```python
from build123d import *

# Parameters (mm, degrees)
F1_DEPTH = 60
F5_D     = 7
F5_DEPTH = 50
F5_TIP   = 2.1030121666
F7_DEPTH = 4.5
F9_DEPTH = 4.5
F10_R    = 1


with BuildPart() as f1:
    # F0 (on Front) → F1 (new body)
    with BuildSketch(Plane.XZ):
        with BuildLine():
            Line((-10, 10), (-10, 0))
            Line((-10, 0), (-7.5, 0))
            Line((-7.5, 0), (-7.5, 5))
            Line((-7.5, 5), (-2.5, 5))
            Line((-2.5, 5), (-2.5, 0))
            Line((-2.5, 0), (2.5, 0))
            Line((2.5, 0), (2.5, 5))
            Line((2.5, 5), (7.5, 5))
            Line((7.5, 5), (7.5, 0))
            Line((7.5, 0), (10, 0))
            Line((10, 0), (10, 10))
            ThreePointArc((10, 10), (0, 20), (-10, 10))
        make_face()
    extrude(amount=-F1_DEPTH)

    # F2 (on Right) → F3 (revolve)
    with BuildSketch(Plane.YZ):
        with BuildLine():
            Line((0, 5), (0, 15))
            ThreePointArc((0, 15), (-5, 10), (0, 5))
        make_face()
    revolve(axis=Axis((0, 0, 10), (0, 0, -1)))

    # F5
    with Locations(Plane(origin=(0, 60, 0), x_dir=(-1, 0, 0), z_dir=(0, 1, 0))):
        with Locations((0, 10)):
            Hole(F5_D / 2, depth=F5_DEPTH)
            with Locations((0, 0, -(F5_DEPTH + F5_TIP / 2))):  # 118° drill point
                Cone(0, F5_D / 2, F5_TIP, mode=Mode.SUBTRACT)

    # F6 (on face) → F7 (join)
    with BuildSketch(Plane.YZ.offset(10)):
        Polygon((45, 0), (60, 0), (48, 10), (45, 10), align=None)
    extrude(amount=F7_DEPTH)

    # F8 (on face) → F9 (join)
    with BuildSketch(Plane(origin=(-10, 0, 0), x_dir=(0, -1, 0), z_dir=(-1, 0, 0))):
        Polygon((-48, 10), (-60, 0), (-45, 0), (-45, 10), align=None)
    extrude(amount=F9_DEPTH)

    # F10
    f10_edges = [f1.edges().sort_by_distance(p)[0] for p in [
        (12.25, 45, 10),
        (12.25, 48, 10),
        (-12.25, 45, 10),
        (-12.25, 48, 10),
    ]]
    fillet(f10_edges, radius=F10_R)


solid = f1.part
```
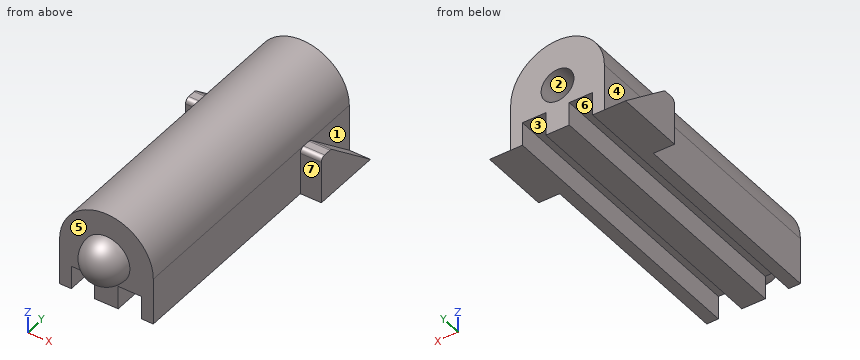
Could you check a few things on this model? Use its own coordinates, in mm. Face numbers are marked on the shaded views. A direction names the side the tool comes from. Coordinates: 2 decimals unless noted, no trailing zeros. Write each loop counter-clockwise with the first axis right and the second up, starting at its lowest first coordinate (ties: lowest second). Pieces come first, ordered by that corner, then holes. Notation, with made-up numbers: (-14.75, 72.5) -> (29.25, 72.5) arc R20 ccw to (29.25, 90.5) -> close; hole circle Ø9 at (48.5, 87.25). An arc over 180 degrees is marked (long way). One line per question, with ' | ' between items. Start each with the question number.
1. Will these pins go through, and if not, where does the flat tip stop? P1, Ø0.5, axis at x = 12, y = 47, coming from the +Z side; P2, Ø2, axis at y = 8, z = 16.5, coming from the +X side; P3, Ø11, axis at y = 23.5, z = 7, coming from the +X side; P4, Ø2, axis at x = 7.5, y = 41, coming from the -Z side.
2. If we section it at D-D (z = 17.25): Please give me the cut outline in (x, y).
3. If we section it at C-C (y = 7): Please give me the cut outline in (x, z).
4. If we section it at A-A (z = 1.5): Please give me the cut outline in (x, y), and give its area (3 significant figures).
5. Please list where these lines run through material, in increasing order: line 1 along X through (y, z) = (16, 4.75); line 2 along X through (y, z) = (48, 10); line 3 along Z through (x, y) = (0, 22.5).
6. If we section it at B-B (y = 15.5): Please give me the cut outline in (x, z), and give its area (3 significant figures).
7. Thinking about a two-plate mould opening in Z: for the marked faces 1, 2 and 3, which applies, pulls with the +Z half, pulls with the -Z half, needs draft (parallel to the pull), parting line crosses it, or undercut?
8. For the marked faces 4, 5, 6 and 7, which set-ups out of +Z, -Z, +X, -X, +Y, -Y let a thin tool reach every point of the face, with its end or its side?
Return value:
1) P1: stops at z = 10 | P2: stops at x = 8.35 | P3: stops at x = 10 | P4: stops at z = 0
2) outline: (-6.89, 0) -> (6.89, 0) -> (6.89, 60) -> (-6.89, 60) -> close
3) outline: (-10, 0) -> (-7.5, 0) -> (-7.5, 5) -> (-2.5, 5) -> (-2.5, 0) -> (2.5, 0) -> (2.5, 5) -> (7.5, 5) -> (7.5, 0) -> (10, 0) -> (10, 10) arc R10 ccw to (-10, 10) -> close
4) outline: (-14.5, 45) -> (-10, 45) -> (-10, 0) -> (-7.5, 0) -> (-7.5, 60) -> (-10, 60) -> (-10, 58.2) -> (-14.5, 58.2) -> close; (-2.5, 0) -> (2.5, 0) -> (2.5, 60) -> (-2.5, 60) -> close; (7.5, 0) -> (10, 0) -> (10, 45) -> (14.5, 45) -> (14.5, 58.2) -> (10, 58.2) -> (10, 60) -> (7.5, 60) -> close | area: 719 mm²
5) line 1: x = -10 to -7.5, -2.5 to 2.5, 7.5 to 10 | line 2: x = -10 to -3.5, 3.5 to 10 | line 3: z = 0 to 6.5, 13.5 to 20
6) outline: (-10, 0) -> (-7.5, 0) -> (-7.5, 5) -> (-2.5, 5) -> (-2.5, 0) -> (2.5, 0) -> (2.5, 5) -> (7.5, 5) -> (7.5, 0) -> (10, 0) -> (10, 10) arc R10 ccw to (-10, 10) -> close; hole circle Ø7 at (0, 10) | area: 269 mm²
7) face 1: needs draft | face 2: undercut | face 3: pulls with the -Z half
8) face 4: +Z, -X, +Y | face 5: -Y | face 6: -Z, +Y, -Y | face 7: +Z, -Z, +X, -Y
